Verification items for the finished model (mm, model axes). Round coordinates to 2 decimals unless told otherwise and drop trailing zeros. Write each loop counter-clockwise with the first axis right and the second up, starting at its lowest first coordinate (ties: lowest second). Pieces come first, ordered by that corner, then holes. Notation, with made-up numbers: M 59,44 L 113,44 A23 ccw 113,65 Z; hole C -17,-19 d11. An arc over 180 degrees is marked long. Answer in a Markdown table with one row per item. Add a question column.
1. Go/stop test with flat-tipped pins: pin 1 Ø5 at (x, y) = (-6.5, 0.5) entering from -Z; pin 2 Ø2 at (x, z) = (-7.5, -3) entering from +Y; pin 3 Ø3 at (x, z) = (-2, 5) entering from +Y; pin 4 Ø4 at (y, z) = (-4.5, 4) entering from +X. Record where each tip stops, or that it passes through.
2. Material ranges on probe 1 along Z at (x, y) = (0, -0.75); probe 2 along Y at (x, z) = (12, 0), recorded low to high.
3. Sectioned sample at D-D on y = -4.5. Record the cut outline in (x, z).
4. Sectioned sample at C-C on y = 2.5. Record the cut outline in (x, z).
5. Draft check along Y on faces 1 (the flat face through (-3, 7.5, -8.2)), 2 (the flat face through (-3, -7.5, -8.2)), 3 (the cylindrical face through (10.269, -1.062, -4.783)). Enter one of: pulls with the +Y half, pulls with the -Y half, needs draft (parallel to the pull), parting line crosses it, or undercut.
6. Sectioned sample at A-A on z = 0. Record the cut outline in (x, y), plus the area to 3 significant figures.
7. Sectioned sample at B-B on x = 0. Record the cut outline in (y, z), plus the area to 3 significant figures.
```python
from build123d import *

# Parameters (mm, degrees)
F0_R     = 13.5
F0_R_2   = 8.5
F1_DEPTH = 7.5
F2_R     = 4.9
F3_DEPTH = 15
F4_SIZE  = 1


with BuildPart() as f1:
    # F0 (on Front) → F1 (new body, symmetric)
    with BuildSketch(Plane.XZ):
        Circle(F0_R)
        Circle(F0_R_2, mode=Mode.SUBTRACT)
    extrude(amount=F1_DEPTH, both=True)

    # F2 (on Right) → F3 (cut, symmetric)
    with BuildSketch(Plane.YZ):
        Circle(F2_R)
    extrude(amount=F3_DEPTH, both=True, mode=Mode.SUBTRACT)

    # F4
    f4_edges = [f1.edges().sort_by_distance(p)[0] for p in [
        (-13.5, -7.5, 0),
        (-13.5, 7.5, 0),
    ]]
    chamfer(f4_edges, length=F4_SIZE)


solid = f1.part
```
Geometry check:
| question | item | result |
|---|---|---|
| 1 | pin 1 | stops at z = -12.89 |
| 1 | pin 2 | stops at y = 7.5 |
| 1 | pin 3 | passes through |
| 1 | pin 4 | stops at x = 13.35 |
| 2 | probe 1 | z = -13.5 to -8.5, 8.5 to 13.5 |
| 2 | probe 2 | y = -7.5 to -4.9, 4.9 to 7.5 |
| 3 | outline | M -13.36,-1.94 A13.5 ccw 13.36,-1.94 L 8.28,-1.94 A8.5 cw -8.28,-1.94 Z; M -13.36,1.94 L -8.28,1.94 A8.5 cw 8.28,1.94 L 13.36,1.94 A13.5 ccw Z |
| 4 | outline | M -12.83,-4.21 A13.5 ccw 12.83,-4.21 L 7.38,-4.21 A8.5 cw -7.38,-4.21 Z; M -12.83,4.21 L -7.38,4.21 A8.5 cw 7.38,4.21 L 12.83,4.21 A13.5 ccw Z |
| 5 | face 1 | pulls with the +Y half |
| 5 | face 2 | pulls with the -Y half |
| 5 | face 3 | undercut |
| 6 | outline | M -13.5,-6.5 L -12.5,-7.5 L -8.5,-7.5 L -8.5,-4.9 L -13.5,-4.9 Z; M -13.5,4.9 L -8.5,4.9 L -8.5,7.5 L -12.5,7.5 L -13.5,6.5 Z; M 8.5,-7.5 L 12.5,-7.5 L 13.5,-6.5 L 13.5,-4.9 L 8.5,-4.9 Z; M 8.5,4.9 L 13.5,4.9 L 13.5,6.5 L 12.5,7.5 L 8.5,7.5 Z |
| 6 | area | 50.0 mm2 |
| 7 | outline | M -7.5,-12.5 L -6.5,-13.5 L 6.5,-13.5 L 7.5,-12.5 L 7.5,-8.5 L -7.5,-8.5 Z; M -7.5,8.5 L 7.5,8.5 L 7.5,12.5 L 6.5,13.5 L -6.5,13.5 L -7.5,12.5 Z |
| 7 | area | 148 mm2 |
